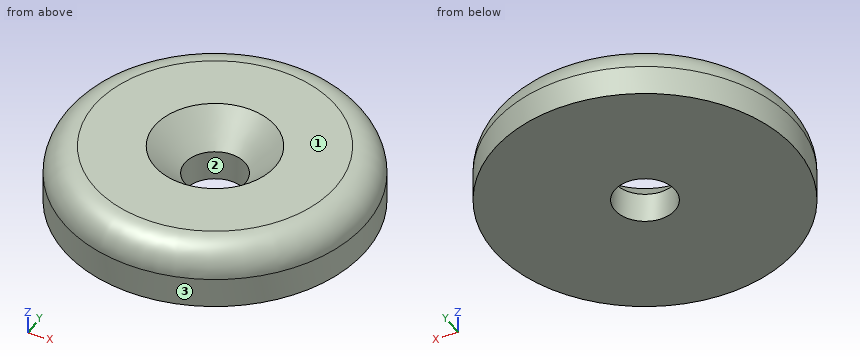
```python
from build123d import *

# Parameters (mm, degrees)
F0_R     = 10
F0_R_2   = 2
F1_DEPTH = 4
F2_R     = 2
F3_SIZE  = 2


with BuildPart() as f1:
    # F0 (on Top) → F1 (new body)
    with BuildSketch(Plane.XY):
        Circle(F0_R)
        Circle(F0_R_2, mode=Mode.SUBTRACT)
    extrude(amount=F1_DEPTH)

    # F2
    f2_edges = [f1.edges().sort_by_distance(p)[0] for p in [
        (-10, 0, 4),
    ]]
    fillet(f2_edges, radius=F2_R)

    # F3
    f3_edges = [f1.edges().sort_by_distance(p)[0] for p in [
        (-2, 0, 4),
    ]]
    chamfer(f3_edges, length=F3_SIZE)


solid = f1.part
```
Input: part model. Units: mm. Frame: model coordinates. Face numbers are marked on the shaded views. Coordinates: 2 decimals unless noted, no trailing zeros. Loops run counter-clockwise (first coordinate to the right, second up) from the corner with the lowest first, then second, coordinate; pieces in that order, holes last. Notation, with made-up numbers: M -12,21 L 10,21 A18 ccw 10,40 Z; hole C 89,-5 d6. An arc over 180 degrees is marked long. Use a Markdown table: item, result. Add a question column.
1) Section A-A, the plane x = 0. Return the cut outline in (y, z), plus the area to 3 significant figures.
2) Pin query (flat end, axial travel): P1, Ø1.5, axis at x = 1, y = -1.5, coming from the +Z side; P2, Ø2.5, axis at x = 0, y = 0, coming from the -Z side. Return the tip coordinate at first contact, or that it passes through.
3) Section D-D, the plane z = 2.45. Return the cut outline in (x, y).
4) Line query: L1, parallel to Y at x = 0, z = 1.4; L2, parallel to X at y = -0.5, z = 1.85; L3, parallel to Y at x = 1.5, z = 1.3. Output: solid intervals per line, ascending. Write a range as from..to.
5) Section C-C, the plane z = 0.45. Return the cut outline in (x, y), plus the area to 3 significant figures.
6) Draft query along X for the marked faces 1, 2 and 3. Return one class per face: +X half, -X half, draft (parallel to the pull), parting line (faces both ways), or undercut.
Answer below:
| question | item | result |
|---|---|---|
| 1 | outline | M -10,0 L -2,0 L -2,2 L -4,4 L -8,4 A2 ccw -10,2 Z; M 2,0 L 10,0 L 10,2 A2 ccw 8,4 L 4,4 L 2,2 Z |
| 1 | area | 58.3 mm2 |
| 2 | P1 | z = 2.55 |
| 2 | P2 | through |
| 3 | outline | C 0,0 d19.9; hole C 0,0 d4.9 |
| 4 | L1 | -10..-2, 2..10 |
| 4 | L2 | -9.99..-1.94, 1.94..9.99 |
| 4 | L3 | -9.89..-1.32, 1.32..9.89 |
| 5 | outline | C 0,0 d20; hole C 0,0 d4 |
| 5 | area | 302 mm2 |
| 6 | face 1 | draft |
| 6 | face 2 | undercut |
| 6 | face 3 | parting line |
